Geometry: see drawing. Coordinates: mm, zero at the bounding-box minimum. A direction names the side the tool comes from. Give positions to 0.01 mm unless a question says otherwise; leave off trailing zeros. Write each loop counter-clockwise with the first axis right and the second up, starting at its lowest first coordinate (ties: lowest second). Pieces come first, ordered by that corner, then holes. Notation, with made-up numbers: (45.5, 79.25) -> (84.5, 79.25) arc R20 ccw to (84.5, 114.25) -> close; hole circle Ø6 at (72.5, 64.25). An arc over 180 degrees is marked (long way). Use one line per item in the form item = value. Start each with the question number.
(1) Draft query along X for the marked faces 3 and 4. Return one class per face: pulls with the +X half, pulls with the -X half, needs draft (parallel to the pull), parting line crosses it, or undercut.
(2) Cut plane A-A, the plane y = 25. Output: boundary loops of the cut face in (x, z).
(3) Cut plane C-C, the plane y = 4. Output: boundary loops of the cut face in (x, z).
(4) First-contact query: P1, Ø10, axis at x = 86, y = 31.5, coming from the +Z side; P2, Ø5, axis at x = 232.5, z = 186.5, coming from the +Y side; P3, Ø10, axis at y = 28, z = 239, coming from the +X side. Flat tips, straight axial feed; report the tip coordinate or a pass-through.
(5) Cut plane B-B, the plane x = 97. Output: boundary loops of the cut face in (y, z), and give its area (3 significant figures).
(6) Material intervals for line 1 along Z through (x, y) = (182, 34); line 2 along Y through (x, z) = (117.5, 23); line 3 along X through (y, z) = (31, 231), sorted ascending. Write a range as from..to.
(7) Set-up query: the marked faces 1 and 2. Return all of +Z, -Z, +X, -X, +Y, -Y with unobstructed straight access to the full face (end or side cutting, diameter ignored); none if empty.
(8) Cut plane D-D, the plane z = 105. Output: boundary loops of the cut face in (x, y), and give its area (3 significant figures).
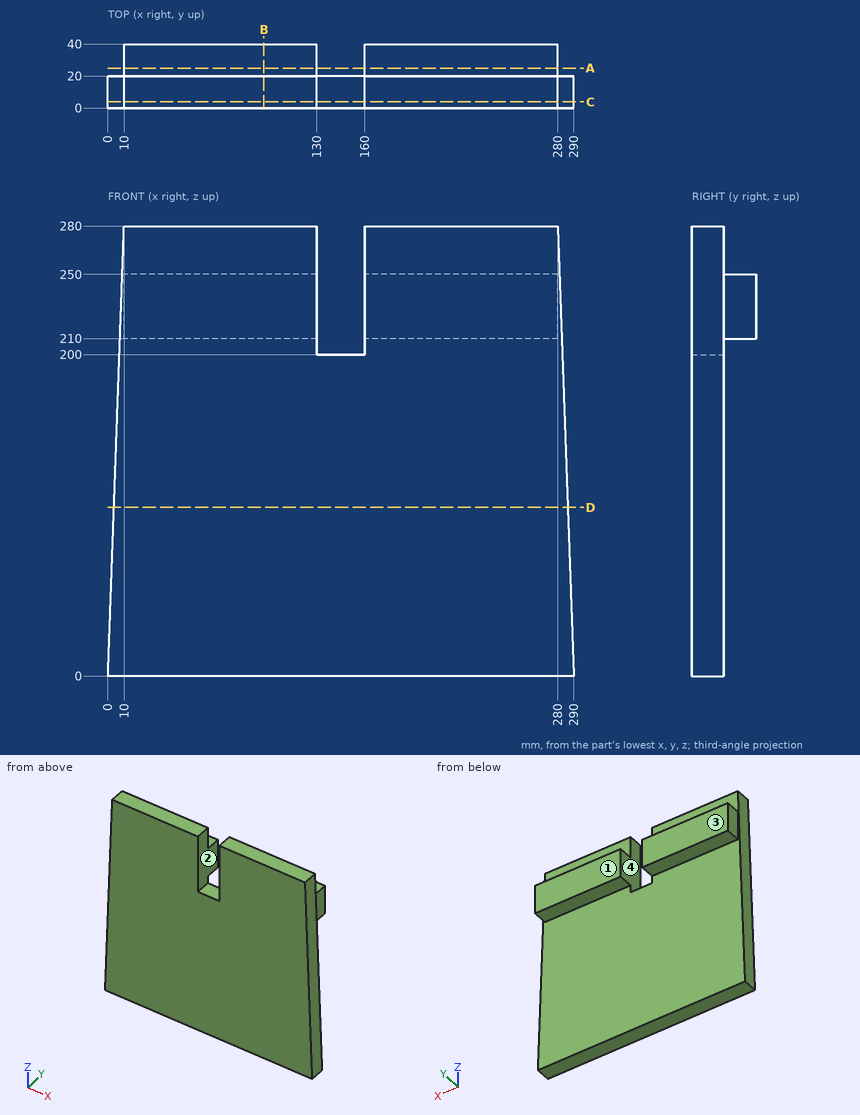
Geometry says:
q1.face_3 = needs draft
q1.face_4 = undercut
q2.outline = (10, 210) -> (130, 210) -> (130, 250) -> (10, 250) -> close; (160, 210) -> (280, 210) -> (280, 250) -> (160, 250) -> close
q3.outline = (0, 0) -> (290, 0) -> (280, 280) -> (160, 280) -> (160, 200) -> (130, 200) -> (130, 280) -> (10, 280) -> close
q4.P1 = 250
q4.P2 = 20
q4.P3 = 280
q5.outline = (0, 0) -> (20, 0) -> (20, 210) -> (40, 210) -> (40, 250) -> (20, 250) -> (20, 280) -> (0, 280) -> close
q5.area = 6,400 mm^2
q6.line_1 = 210..250
q6.line_2 = 0..20
q6.line_3 = 10..130, 160..280
q7.face_1 = +Z, -Z, +X, -X, +Y
q7.face_2 = +Z, +Y, -Y
q8.outline = (3.75, 0) -> (286.25, 0) -> (286.25, 20) -> (3.75, 20) -> close
q8.area = 5,650 mm^2
